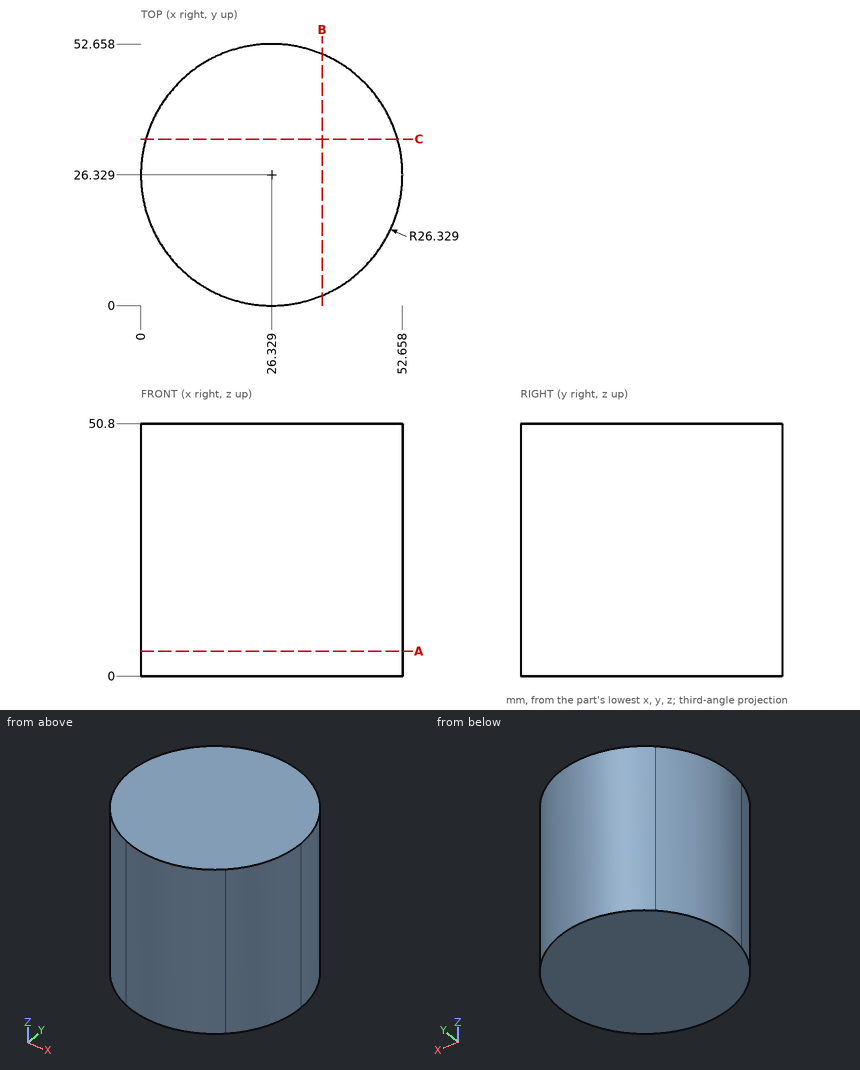
Geometry: see drawing. Coordinates: mm, zero at the bounding-box minimum. Coordinates: 2 decimals unless noted, no trailing zeros. Order: outer loops, then holes, each group sorted by start corner. A loop starts at its lowest first (then second) coordinate and runs counter-clockwise, first axis right, second up. Notation, with made-up numbers: (13, 74) -> (22, 74) arc R6 cw to (22, 81) -> close; hole circle Ø9 at (13, 55). An arc over 180 degrees is marked (long way). Write each question's results on one line, items separated by ' | '. Start each with the question number.
1) Material intervals for line 1 along X through (y, z) = (27, 41.5); line 2 along X through (y, z) = (26, 39); line 3 along Y through (x, z) = (11, 39.5) (1 decimal), sorted ascending.
2) Cut plane A-A, the plane z = 5. Output: boundary loops of the cut face in (x, y).
3) Cut plane B-B, the plane x = 36.5. Output: boundary loops of the cut face in (y, z).
4) Cut plane C-C, the plane y = 33.5. Output: boundary loops of the cut face in (x, z) (1 decimal), and give its area (3 significant figures).
5) First-contact query: pin 1 (12 mm diameter, centred on y = 46, z = 22.5, fed in from -X); pin 2 (1 mm diameter, centred on x = 46, z = 22.5, fed in from -Y); pin 3 (5 mm diameter, centred on x = 11.5, z = 37, fed in from -Y) (1 decimal). Flat tips, straight axial feed; report the tip coordinate or a pass-through.
Checks:
1) line 1: 0.01 to 52.65 | line 2: 0 to 52.66 | line 3: 4.9 to 47.7
2) outline: (0.57, 20.89) arc R26.33 ccw to (16.19, 2.03) arc R26.33 ccw to (43.61, 6.47) arc R26.33 ccw to (52.66, 26.33) arc R26.33 ccw to (9.05, 46.19) arc R26.33 ccw to start
3) outline: (2.04, 0) -> (50.61, 0) -> (50.61, 50.8) -> (2.04, 50.8) -> close
4) outline: (1, 0) -> (51.7, 0) -> (51.7, 50.8) -> (1, 50.8) -> close | area: 2,570 mm^2
5) pin 1: x = 3.83 | pin 2: y = 8.28 | pin 3: y = 3.1
